Work out the finished part from the listing and answer in its coordinate system (mm). A direction names the side the tool comes from. Round coordinates to 2 decimals unless told otherwise and drop trailing zeros. Order: outer loops, then holes, each group sorted by start corner. A loop starts at its lowest first (then second) coordinate and runs counter-clockwise, first axis right, second up.
Autodesk Inventor part; units mm, degrees
ref_plane "Arbeitsebene1" through (0, 0, 2.5) normal (0, 0, 1) x (1, 0, 0)
ref_plane "YZ Plane" through (0, 0, 0) normal (1, 0, 0) x (0, 1, 0)
ref_plane "XZ Plane" through (0, 0, 0) normal (0, 1, 0) x (-1, 0, 0)
sketch "Skizze1" plane through (0, 0, 0) normal (0, 0, 1) x (1, 0, 0)
  circle A0 centre (0, 0) radius 3
  dimension "d2" = 6
extrude "Extrusion1" add sketch "Skizze1" against normal blind 70
sketch "Skizze2" plane through (0, 0, 0) normal (0, 0, 1) x (1, 0, 0)
  circle A0 centre (0, 0) radius 3
  circle A1 centre (0, 0) radius 3
  dimension "d36" = 6
extrude "Extrusion2" add sketch "Skizze2" along normal blind 1
sketch "Skizze3" plane through (0, 0, 1) normal (0, 0, 1) x (1, 0, 0)
  circle A0 centre (0, 0) radius 3
  circle A1 centre (0, 0) radius 3
  dimension "d28" = 6
extrude "Extrusion3" add sketch "Skizze3" along normal blind 8
ref_plane "Arbeitsebene1" through (0, 0, 2.5) normal (0, 0, 1) x (1, 0, 0)
sketch "Skizze4" plane through (0, 0, 2.5) normal (0, 0, 1) x (1, 0, 0)
  circle A0 centre (0, 0) radius 3
extrude "Extrusion4" [suppressed]
hole "Bohrung1" at (0, 0, 9) direction (0, 0, -1) diameter 3 depth 23
chamfer "Fase1" distance 0.1 angle 45 1 edges at (0, 1.5, 9)
sketch "Skizze5" plane through (0, 0, 9) normal (0, 0, 1) x (1, 0, 0)
  circle A0 centre (0, 0) radius 3
  line L0 (-3.5, -0.15) -> (3.5, -0.15)
  line L1 (3.5, -0.15) -> (3.5, 0.15)
  line L2 (3.5, 0.15) -> (-3.5, 0.15)
  line L3 (-3.5, 0.15) -> (-3.5, -0.15)
  line L4 (-3.5, -0.15) -> (3.5, 0.15) construction
  line L5 (3.5, -0.15) -> (-3.5, 0.15) construction
  line L6 (-0.15, -3.5) -> (0.15, -3.5)
  line L7 (0.15, -3.5) -> (0.15, 3.5)
  line L8 (0.15, 3.5) -> (-0.15, 3.5)
  line L9 (-0.15, 3.5) -> (-0.15, -3.5)
  line L10 (-0.15, -3.5) -> (0.15, 3.5) construction
  line L11 (0.15, -3.5) -> (-0.15, 3.5) construction
extrude "Extrusion5" cut sketch "Skizze5" against normal up to surface (8 mm away) contours A0 L0 L7 L2 | A0 L2 L1 L0 | L7 L2 L9 A0 | A0 L9 L8 L7 | L7 L0 L9 L2 | L7 L6 L9 A0 | A0 L9 L0 L7 | L9 L0 A0 L2 | A0 L0 L3 L2
sketch "Skizze6" plane through (0, 0, 0) normal (0, 1, 0) x (-1, 0, 0)
  line L0 (0, 0) -> (-2, 0)
  line L1 (0, -1.8) -> (0, 10.8)
  circle A0 centre (-3, 8) radius 1
  line L2 (-0.15, 9) -> (-2.9962, 9)
  dimension "d33" = 3
  dimension "d34" = 2
  dimension "d35" = 1
revolve "Umdrehung1" cut sketch "Skizze6" angle 360 about axis through (0, 0, -10) along (0, 0, 1)
equation "\"d2\" = LowerDiameter"
equation "\"d0\" = LowerLength"
equation "\"d36\" = SealingRingDiameter"
equation "\"d3\" = SealingRingThickness"
equation "\"d28\" = UpperDiameter"
equation "\"d5\" = UpperLength"
equation "\"d9\" = DrillDiameter"
equation "\"d14\" = DrillDepth"
equation "\"UpperDiameter\" = 6"
equation "\"LowerDiameter\" = 6"
equation "\"UpperLength\" = 8"
equation "\"LowerLength\" = 70"
equation "\"SealingRingDiameter\" = 6"
equation "\"SealingRingThickness\" = 1"
equation "\"DrillDiameter\" = 3"
equation "\"DrillDepth\" = 23"
properties part number "specimen_holder_rod_6mm" material "Edelstahl"
Item 1: A tool of negligible diameter and unlimited length cuts with its end or side. For faces 4 (the face through (-0.15, 2, 4)), 5 (the face through (-2, 0.15, 4)), 6 (the face through (0, 0, -14)), from which of +Z, -Z, +X, -X, +Y, -Y can it reach the whole face along a straight path? Write none if from no direction.
Item 2: Find section C-C (z = -62). Write down the section's boundary in (x, y), plus the area to 3 significant figures.
Item 3: For a pull along Y with two mould halves and no side action, classify faces 1 (the face through (-0.45, -1.43, -2.71)), 2 (the face through (0.15, -2, 4)), 3 (the face through (2.86, -0.9, -32.04)) as released by +Y, released by -Y, zero draft, split by the parting line, or undercut.
Item 4: Given pin 1 (1.7 mm diameter, centred on y = 2.5, z = 5, fed in from +X); pin 2 (0.5 mm diameter, centred on y = -2, z = 7, fed in from +X); pin 3 (1.2 mm diameter, centred on x = 2.5, z = 7, fed in from +Y); pin 4 (2.5 mm diameter, centred on x = -0.5, y = 0.5, fed in from +Z), each flat-ended and moving along its own axis, determine where each tip first touches the part or whether it passes through.
Item 5: Find section A-A (z = 2). Write down the section's boundary in (x, y).
Item 6: Find section B-B (z = -9). Write down the section's boundary in (x, y), plus the area to 3 significant figures.
Item 7: Find the intervals of material crossed by line 1 along Y through (x, z) = (0, -6); line 2 along Z through (x, y) = (-0.45, -0.9), in increasing order.
Model answer:
1. face 4: +Z, +Y, -Y
1. face 5: +Z, +X, -X
1. face 6: +Z
2. outline: circle Ø6 at (0, 0)
2. area: 28.3 mm2
3. face 1: undercut
3. face 2: zero draft
3. face 3: split by the parting line
4. pin 1: stops at x = 2.51
4. pin 2: stops at x = 2.44
4. pin 3: stops at y = 2.32
4. pin 4: stops at z = 9
5. outline: (-3, -0.15) arc R3 ccw to (-0.15, -3) - (-0.15, -1.49) arc R1.5 cw to (-1.49, -0.15) - close; (-3, 0.15) - (-1.49, 0.15) arc R1.5 cw to (-0.15, 1.49) - (-0.15, 3) arc R3 ccw to start; (0.15, -3) arc R3 ccw to (3, -0.15) - (1.49, -0.15) arc R1.5 cw to (0.15, -1.49) - close; (0.15, 1.49) arc R1.5 cw to (1.49, 0.15) - (3, 0.15) arc R3 ccw to (0.15, 3) - close
6. outline: circle Ø6 at (0, 0); hole circle Ø3 at (0, 0)
6. area: 21.2 mm2
7. line 1: y = -3 to -1.5, 1.5 to 3
7. line 2: z = -70 to -14
